```python
from build123d import *

# Parameters (mm, degrees)
SKETCH1_R           = 6.35
SKETCH1_R_2         = 3.175
BOSS_EXTRUDE1_DEPTH = 59.69
CUT_EXTRUDE1_START  = 1.905
SKETCH2_R           = 6.35
SKETCH2_R_2         = 5.715
CUT_EXTRUDE1_DEPTH  = 0.9906
SKETCH3_R           = 6.35
BOSS_EXTRUDE2_DEPTH = 1.064499902


with BuildPart() as part:
    # Sketch1 → Boss-Extrude1 (new body, symmetric)
    with BuildSketch(Plane(origin=(0, 0, 0), x_dir=(1, 0, 0), z_dir=(0, 1, 0))):
        Circle(SKETCH1_R)
        Circle(SKETCH1_R_2, mode=Mode.SUBTRACT)
        Circle(SKETCH1_R_2)
    extrude(amount=BOSS_EXTRUDE1_DEPTH, both=True)

    # Sketch2 → Cut-Extrude1 (cut)
    with BuildSketch(Plane(origin=(0, -59.69, 0), x_dir=(1, 0, 0), z_dir=(0, 1, 0)).offset(CUT_EXTRUDE1_START)):
        Circle(SKETCH2_R)
        Circle(SKETCH2_R_2, mode=Mode.SUBTRACT)
    cut_extrude1 = extrude(amount=-CUT_EXTRUDE1_DEPTH, mode=Mode.SUBTRACT)

    # Mirror1: Cut-Extrude1 across plane
    add(cut_extrude1.mirror(Plane.ZX), mode=Mode.SUBTRACT)

    # Sketch3 → Boss-Extrude2 (add)
    with BuildSketch(Plane(origin=(0, 59.69, 0), x_dir=(1, 0, 0), z_dir=(0, 1, 0))):
        Circle(SKETCH3_R)
    boss_extrude2 = extrude(amount=BOSS_EXTRUDE2_DEPTH)

    # Mirror2: Boss-Extrude2 across plane
    add(boss_extrude2.mirror(Plane.ZX))


solid = part.part
```
Build history of the part. All positions in model axes, mm. A direction names the side the tool comes from. Round coordinates to 2 decimals unless told otherwise and drop trailing zeros. Write each loop counter-clockwise with the first axis right and the second up, starting at its lowest first coordinate (ties: lowest second). Pieces come first, ordered by that corner, then holes.
1) Band-saw the part on B-B, the plane z = 4.25. List the corners of the cut face in (x, y) (1 decimal).
2) Drill centre lines: probe 1 along Y at (x, z) = (-3, -5.5) (1 decimal); probe 2 along X at (y, z) = (30, -0.5); probe 3 along Z at (x, y) = (2.75, 6). Where is each one in solid material? Low to high.
3) Band-saw the part on A-A, the plane x = -2. List the corners of the cut face in (y, z) (1 decimal), and give its area (3 significant figures).
4) Pin check, flat tips, straight feed: pin 1 (2 mm diameter, centred on x = 3.5, y = 2, fed in from +Z); pin 2 (1.5 mm diameter, centred on y = 27.5, z = -3, fed in from -X); pin 3 (5 mm diameter, centred on x = -4, y = 9, fed in from +Z). Stop position of each tip, or through.
5) Mould opens along Y. For faces 3 (the flat face through (-6, 58.776, -1)), 4 (the flat face through (0, -60.754, 0)), 5 (the flat face through (-6, -58.776, -1)), 6 (the cylindrical face through (-1.38, 0.81, 6.2)) say: +Y half, -Y half, draft (parallel to the pull), parting line (faces both ways), or undercut.
6) Band-saw the part on C-C, the plane y = 25.5. List the corners of the cut face in (x, z), and give its area (3 significant figures).
7) 3-axis set-ups, long thin cutter, end or side, ignore diameter. For faces 1 (the cylindrical face through (-1.38, 59.78, 6.2)), 2 (the flat face through (-6, -57.785, -1)): which of +Z, -Z, +X, -X, +Y, -Y reach the whole face in a straight line?
Ans:
1. outline: (-4.7, -60.8) - (4.7, -60.8) - (4.7, -58.8) - (3.8, -58.8) - (3.8, -57.8) - (4.7, -57.8) - (4.7, 57.8) - (3.8, 57.8) - (3.8, 58.8) - (4.7, 58.8) - (4.7, 60.8) - (-4.7, 60.8) - (-4.7, 58.8) - (-3.8, 58.8) - (-3.8, 57.8) - (-4.7, 57.8) - (-4.7, -57.8) - (-3.8, -57.8) - (-3.8, -58.8) - (-4.7, -58.8) - close
2. probe 1: y = -60.8 to -58.8, -57.8 to 57.8, 58.8 to 60.8
2. probe 2: x = -6.33 to 6.33
2. probe 3: z = -5.72 to 5.72
3. outline: (-60.8, -6) - (-58.8, -6) - (-58.8, -5.4) - (-57.8, -5.4) - (-57.8, -6) - (57.8, -6) - (57.8, -5.4) - (58.8, -5.4) - (58.8, -6) - (60.8, -6) - (60.8, 6) - (58.8, 6) - (58.8, 5.4) - (57.8, 5.4) - (57.8, 6) - (-57.8, 6) - (-57.8, 5.4) - (-58.8, 5.4) - (-58.8, 6) - (-60.8, 6) - close
3. area: 1,460 mm2
4. pin 1: stops at z = 5.84
4. pin 2: stops at x = -5.94
4. pin 3: stops at z = 6.17
5. face 3: undercut
5. face 4: -Y half
5. face 5: undercut
5. face 6: draft
6. outline: circle Ø12.7 at (0, 0)
6. area: 127 mm2
7. face 1: +Y, -Y
7. face 2: none
